Source: three-view drawing plus pictorial views. Frame: mm from the lowest corner of the part. Coordinates: 2 decimals unless noted, no trailing zeros. Order: outer loops, then holes, each group sorted by start corner. A loop starts at its lowest first (then second) coordinate and runs counter-clockwise, first axis right, second up. Notation, with made-up numbers: (12.25, 3) - (17.25, 3) arc R24 cw to (17.25, 42) - close; hole circle Ø8 at (-14.5, -27.75). An arc over 180 degrees is marked (long way). One line per question, with ' | ' between items.
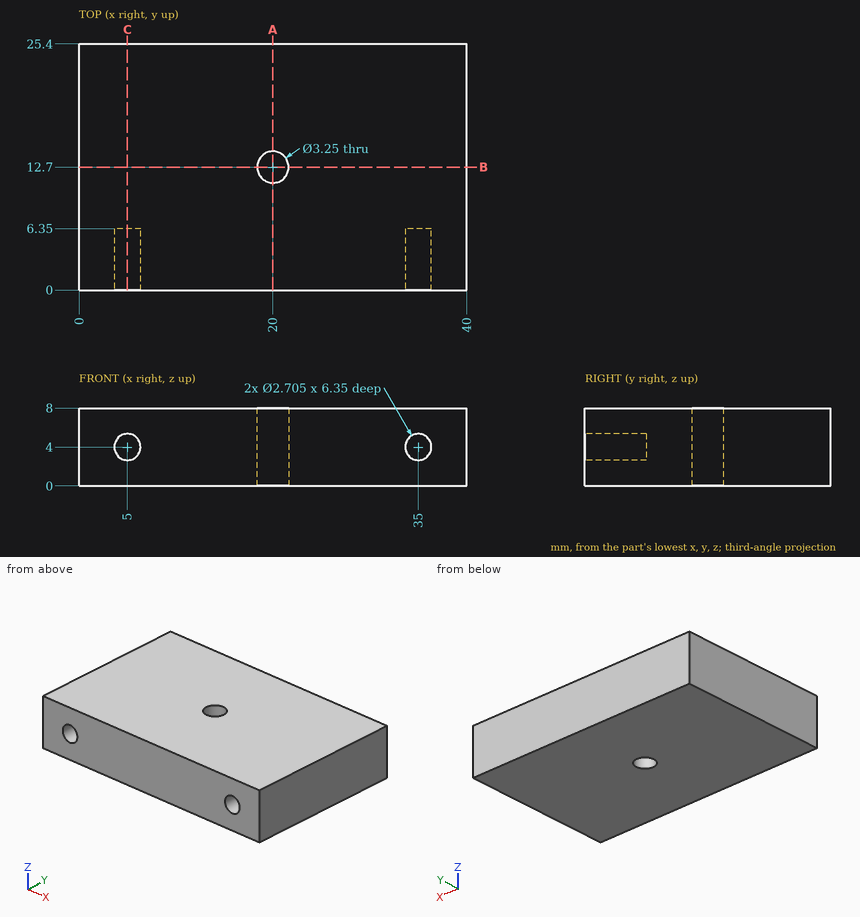
(1) Cut plane C-C (x = 5). Return the cut outline in (y, z), and give its area (3 significant figures).
Taken from the geometry:
outline: (0, 0) - (25.4, 0) - (25.4, 8) - (0, 8) - (0, 5.35) - (6.35, 5.35) - (6.35, 2.65) - (0, 2.65) - close | area: 186 mm²
(2) Cut plane A-A (x = 20). Return the cut outline in (y, z) (3 decimals), and give its area (3 significant figures).
Taken from the geometry:
outline: (0, 0) - (11.075, 0) - (11.075, 8) - (0, 8) - close; (14.325, 0) - (25.4, 0) - (25.4, 8) - (14.325, 8) - close | area: 177 mm²
(3) Pin query (flat end, axial travel): P1, Ø2.5, axis at x = 5, z = 4, coming from the -Y side. Return the tip coordinate at first contact, or that it passes through.
Taken from the geometry:
P1: stops at y = 6.35
(4) Cut plane B-B (y = 12.7). Return the cut outline in (x, z) (3 decimals), and give its area (3 significant figures).
Taken from the geometry:
outline: (0, 0) - (18.375, 0) - (18.375, 8) - (0, 8) - close; (21.625, 0) - (40, 0) - (40, 8) - (21.625, 8) - close | area: 294 mm²
(5) Material intervals for L1, parallel to Z at x = 5, y = 2.75; L2, parallel to Y at x = 20.5, z = 6.25, sorted ascending. Write a range as from..to.
Taken from the geometry:
L1: z = 0..2.65, 5.35..8 | L2: y = 0..11.15, 14.25..25.4
